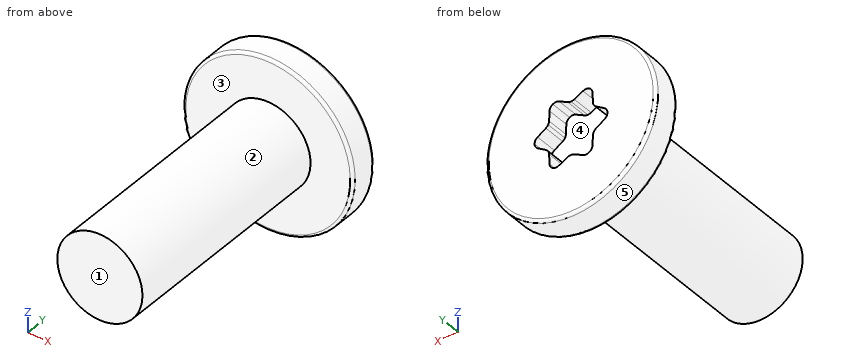
from build123d import *

# Parameters (mm, degrees)
FILLET1_R          = 0.1
SKETCH2_R          = 0.93
CUT_EXTRUDE1_DEPTH = 0.8


with BuildPart() as part:
    # Sketch1 → Revolve1 (revolve)
    with BuildSketch(Plane(origin=(0, 0, 0), x_dir=(0, 0, -1), z_dir=(1, 0, 0))):
        Polygon((0, 0), (0, -9), (1.5, -9), (1.5, -1), (3, -1), (3, 0), align=None)
    revolve(axis=Axis((0, 0, 0), (0, 1, 0)))

    # Fillet1
    fillet1_edges = [part.edges().sort_by_distance(p)[0] for p in [
        (0, 0, 3),
        (0, -1, 3),
    ]]
    fillet(fillet1_edges, radius=FILLET1_R)

    # Sketch2 → Cut-Extrude1 (cut)
    with BuildSketch(Plane(origin=(0, 0, 0), x_dir=(1, 0, 0), z_dir=(0, 1, 0))):
        Circle(SKETCH2_R)
        with BuildLine():
            ThreePointArc((0.757286248, 0.923570431), (0.724160575, 1.032923804), (0.6425, 1.112842644))
            ThreePointArc((0.6425, 1.112842644), (0.532457967, 1.143603357), (0.421192331, 1.117614344))
            Line((0.421192331, 1.117614344), (0.115551814, 0.958307018))
            ThreePointArc((0.115551814, 0.958307018), (0.059484261, 0.937179855), (0, 0.93))
            ThreePointArc((0, 0.93), (0.465000014, 0.805403617), (0.805403642, 0.464999972))
            ThreePointArc((0.805403642, 0.464999972), (0.781879437, 0.520104793), (0.772142315, 0.579224316))
            Line((0.772142315, 0.579224316), (0.757286248, 0.923570431))
        make_face()
        with BuildLine():
            ThreePointArc((-0.6425, 1.112842644), (-0.724160575, 1.032923804), (-0.757286248, 0.923570431))
            Line((-0.757286248, 0.923570431), (-0.772142315, 0.579224316))
            ThreePointArc((-0.772142315, 0.579224316), (-0.781879432, 0.52010481), (-0.805403624, 0.465000003))
            ThreePointArc((-0.805403624, 0.465000003), (-0.464999999, 0.805403626), (0, 0.93))
            ThreePointArc((0, 0.93), (-0.059484261, 0.937179855), (-0.115551814, 0.958307018))
            Line((-0.115551814, 0.958307018), (-0.421192331, 1.117614344))
            ThreePointArc((-0.421192331, 1.117614344), (-0.532457967, 1.143603357), (-0.6425, 1.112842644))
        make_face()
        with BuildLine():
            ThreePointArc((-0.805403626, -0.464999999), (-0.93, 2e-09), (-0.805403624, 0.465000003))
            ThreePointArc((-0.805403624, 0.465000003), (-0.841363692, 0.417075048), (-0.887694129, 0.379082702))
            Line((-0.887694129, 0.379082702), (-1.178478579, 0.194043914))
            ThreePointArc((-1.178478579, 0.194043914), (-1.256618542, 0.110679553), (-1.285, 0))
            ThreePointArc((-1.285, 0), (-1.256618542, -0.110679553), (-1.178478579, -0.194043914))
            Line((-1.178478579, -0.194043914), (-0.887694129, -0.379082702))
            ThreePointArc((-0.887694129, -0.379082702), (-0.841363693, -0.417075046), (-0.805403626, -0.464999999))
        make_face()
        with BuildLine():
            ThreePointArc((-3e-09, -0.93), (-0.465000002, -0.805403625), (-0.805403626, -0.464999999))
            ThreePointArc((-0.805403626, -0.464999999), (-0.781879432, -0.520104808), (-0.772142315, -0.579224316))
            Line((-0.772142315, -0.579224316), (-0.757286248, -0.923570431))
            ThreePointArc((-0.757286248, -0.923570431), (-0.724160575, -1.032923804), (-0.6425, -1.112842644))
            ThreePointArc((-0.6425, -1.112842644), (-0.532457967, -1.143603357), (-0.421192331, -1.117614344))
            Line((-0.421192331, -1.117614344), (-0.115551814, -0.958307018))
            ThreePointArc((-0.115551814, -0.958307018), (-0.059484262, -0.937179855), (-3e-09, -0.93))
        make_face()
        with BuildLine():
            ThreePointArc((0.805403624, -0.465000003), (0.464999998, -0.805403627), (-3e-09, -0.93))
            ThreePointArc((-3e-09, -0.93), (0.059484259, -0.937179855), (0.115551814, -0.958307018))
            Line((0.115551814, -0.958307018), (0.421192331, -1.117614344))
            ThreePointArc((0.421192331, -1.117614344), (0.532457967, -1.143603357), (0.6425, -1.112842644))
            ThreePointArc((0.6425, -1.112842644), (0.724160575, -1.032923804), (0.757286248, -0.923570431))
            Line((0.757286248, -0.923570431), (0.772142315, -0.579224316))
            ThreePointArc((0.772142315, -0.579224316), (0.781879432, -0.52010481), (0.805403624, -0.465000003))
        make_face()
        with BuildLine():
            ThreePointArc((1.178478579, -0.194043914), (1.256618542, -0.110679553), (1.285, 0))
            ThreePointArc((1.285, 0), (1.256618542, 0.110679553), (1.178478579, 0.194043914))
            Line((1.178478579, 0.194043914), (0.887694129, 0.379082702))
            ThreePointArc((0.887694129, 0.379082702), (0.841363704, 0.417075035), (0.805403642, 0.464999972))
            ThreePointArc((0.805403642, 0.464999972), (0.898311023, 0.240701696), (0.93, 0))
            ThreePointArc((0.93, 0), (0.898311018, -0.240701713), (0.805403624, -0.465000003))
            ThreePointArc((0.805403624, -0.465000003), (0.841363692, -0.417075048), (0.887694129, -0.379082702))
            Line((0.887694129, -0.379082702), (1.178478579, -0.194043914))
        make_face()
    extrude(amount=-CUT_EXTRUDE1_DEPTH, mode=Mode.SUBTRACT)


solid = part.part
The listing builds one solid part. Answer for the finished solid, in the listing's coordinates (mm). Face numbers are marked on the shaded views. A direction names the side the tool comes from. Give positions to 0.01 mm unless a question says otherwise; leave off trailing zeros. Order: outer loops, then holes, each group sorted by start corner. A loop starts at its lowest first (then second) coordinate and runs counter-clockwise, first axis right, second up. Notation, with made-up numbers: (58.5, -2) - (84.5, -2) arc R21 cw to (84.5, 10) - close; hole circle Ø8 at (21, 47.25). An arc over 180 degrees is marked (long way). One line per item, written item: value. Start each with the question number.
1) A tool of negligible diameter and unlimited length cuts with its end or side. For the marked faces 1 and 2, from which of +Z, -Z, +X, -X, +Y, -Y can it reach the whole face along a straight path? Write none if from no direction.
2) Given pin 1 Ø1 at (y, z) = (-1, 1) entering from +X; pin 2 Ø3 at (y, z) = (-8, 0) entering from -X; pin 3 Ø2 at (y, z) = (-4, -2) entering from +X, each flat-ended and moving along its own axis, determine where each tip first touches the part or whether it passes through.
3) A cutting plane is placed at A-A on y = -2. Give the vertices of the cut face in (x, z).
4) Find the intervals of material crossed by L1, parallel to Z at x = -1, y = -5; L2, parallel to Y at x = 2, z = -0.5; L3, parallel to Y at x = 0.5, z = 1, in increasing order.
5) The mould has two halves that part along Z. Classify the marked faces 3, 4 and 5: released by +Z, released by -Z, zero draft, split by the parting line, or undercut.
Answer sheet:
1. face 1: +Z, -Z, +X, -X, -Y
1. face 2: -Y
2. pin 1: stops at x = 2.96
2. pin 2: stops at x = -1.5
2. pin 3: stops at x = 1.12
3. outline: circle Ø3 at (0, 0)
4. L1: z = -1.12 to 1.12
4. L2: y = -1 to 0
4. L3: y = -9 to -0.8
5. face 3: zero draft
5. face 4: undercut
5. face 5: split by the parting line
